Autodesk Inventor part; units mm, degrees
ref_plane "YZ Plane" through (0, 0, 0) normal (1, 0, 0) x (0, 1, 0)
ref_plane "XZ Plane" through (0, 0, 0) normal (0, 1, 0) x (-1, 0, 0)
ref_plane "XY Plane" through (0, 0, 0) normal (0, 0, 1) x (1, 0, 0)
sketch "Sketch8" plane through (0, 0, 0) normal (0, 0, 1) x (1, 0, 0)
  circle A0 centre (0, 0) radius 6
  dimension "d35" = 12
extrude "Extrusion4" add sketch "Sketch8" along normal blind 7
sketch "Sketch9" plane through (0, 0, 7) normal (0, 0, 1) x (1, 0, 0)
  line L0 (-2.5, 2.5) -> (2.5, 2.5)
  line L1 (2.5, 2.5) -> (2.5, -2.5)
  line L2 (2.5, -2.5) -> (-2.5, -2.5)
  line L3 (-2.5, -2.5) -> (-2.5, 2.5)
  point P0 (0, 0)
  point P1 (0, 0)
  dimension "d38" = 5
  dimension "d39" = 5
  dimension "d40" = 2.5
  dimension "d41" = 2.5
sketch "Sketch10" plane through (0, 0, 0) normal (0, 0, -1) x (-1, 0, 0)
  line L0 (-3, 3) -> (3, 3)
  line L1 (3, 3) -> (3, -3)
  line L2 (3, -3) -> (-3, -3)
  line L3 (-3, -3) -> (-3, 3)
  point P0 (0, 0)
  dimension "d42" = 6
  dimension "d43" = 6
  dimension "d44" = 3
  dimension "d45" = 3
loft "Loft3" cut profiles "Sketch9", "Sketch10"
sketch "Sketch11" plane through (0, 0, 7) normal (0, 0, 1) x (1, 0, 0)
  circle A0 centre (0, 0) radius 6
extrude "Extrusion5" add sketch "Sketch11" along normal blind 2
sketch "Sketch12" plane through (0, 0, 9) normal (0, 0, 1) x (1, 0, 0)
  circle A0 centre (0, 0) radius 1.5
  dimension "d52" = 3
extrude "Extrusion6" add sketch "Sketch12" along normal blind 8
properties part number "Input Connection"
Could you check a few things on this model? Use its own coordinates, in mm. A direction names the side the tool comes from. Round coordinates to 2 decimals unless told otherwise and drop trailing zeros. Order: outer loops, then holes, each group sorted by start corner. A loop starts at its lowest first (then second) coordinate and runs counter-clockwise, first axis right, second up. Notation, with made-up numbers: M -25.75,7.25 L -20.75,7.25 A25 cw -20.75,19.25 Z; hole C -26,-11.5 d1. An arc over 180 degrees is marked long. One line per item, written item: value.
(1) Which directions (+Z, -Z, +X, -X, +Y, -Y) give clear straight access to the entire face, cutting with the end or side of a thin tool? Please do faces 1 (the flat face through (0, 0, 7)), 2 (the flat face through (0, -4, 0)), 3 (the flat face through (1.2, -1.2, 9)).
Ans:
face 1: -Z
face 2: -Z, +X, -X, +Y, -Y
face 3: +Z
(2) Imagine slicing it at D-D (z = 8). Write out the boundary of the cut face in (x, y), and give its area (3 significant figures).
Ans:
outline: C 0,0 d12
area: 113 mm^2
(3) I'm going to push flat-ended pins straight in: P1, Ø1.5, axis at y = 1.5, z = 2, coming from the +X side; P2, Ø2.5, axis at x = 1, y = 0.5, coming from the -Z side; P3, Ø5, axis at x = -3, z = 3, coming from the -Y side. Where does each tip first touch, or does it pass through?
Ans:
P1: stops at x = 5.95
P2: stops at z = 7
P3: stops at y = -5.98
(4) Imagine slicing it at C-C (x = 3.75). Write out the boundary of the cut face in (y, z).
Ans:
outline: M -4.68,0 L 4.68,0 L 4.68,9 L -4.68,9 Z
(5) I need wall thicknesses on line 1 along Z through (x, y) = (1, -5.25); line 2 along Z through (x, y) = (-1.5, -1.5); line 3 along X through (y, z) = (-0.25, 1.75) (3 decimals). Which ranges of each line are inside material? Lowest first, please. Write a range as from..to.
Ans:
line 1: z = 0..9
line 2: z = 7..9
line 3: x = -5.995..-2.875, 2.875..5.995
(6) Imagine slicing it at A-A (z = 15). Write out the boundary of the cut face in (x, y).
Ans:
outline: C 0,0 d3
(7) Imagine slicing it at B-B (y = -4). Write out the boundary of the cut face in (x, z).
Ans:
outline: M -4.47,0 L 4.47,0 L 4.47,9 L -4.47,9 Z
